```python
from build123d import *

# Parameters (mm, degrees)
F1_DEPTH = 6.35
F0_R     = 12.7
F2_DEPTH = 12.7
F3_DEPTH = 3.175
F4_R     = 3.175
F5_DEPTH = 180.976


with BuildPart() as f1:
    # F0 (on Top) → F1 (new body, symmetric)
    with BuildSketch(Plane.XY):
        with BuildLine():
            ThreePointArc((0, -31.75), (-31.75, 0), (0, 31.75))
            Line((0, 31.75), (0, 44.45))
            Line((0, 44.45), (-12.7, 44.45))
            Line((-12.7, 44.45), (-12.7, 31.75))
            Line((-12.7, 31.75), (-19.05, 31.75))
            ThreePointArc((-19.05, 31.75), (-37.291778, 15.423719), (-61.051302, 9.525))
            Line((-61.051302, 9.525), (-143.102955, 9.525))
            ThreePointArc((-143.102955, 9.525), (-150.147647, 10.521469), (-156.639598, 13.432692))
            ThreePointArc((-156.639598, 13.432692), (-151.201718, 7.671595), (-149.225, 0))
            ThreePointArc((-149.225, 0), (-151.201718, -7.671595), (-156.639598, -13.432692))
            ThreePointArc((-156.639598, -13.432692), (-150.147647, -10.521469), (-143.102955, -9.525))
            Line((-143.102955, -9.525), (-61.051302, -9.525))
            ThreePointArc((-61.051302, -9.525), (-37.291778, -15.423719), (-19.05, -31.75))
            Line((-19.05, -31.75), (-12.7, -31.75))
            Line((-12.7, -31.75), (-12.7, -44.45))
            Line((-12.7, -44.45), (0, -44.45))
            Line((0, -44.45), (0, -31.75))
        make_face()
        with BuildLine():
            ThreePointArc((-127, -6.35), (-133.35, 0), (-127, 6.35))
            Line((-127, 6.35), (-50.8, 6.35))
            ThreePointArc((-50.8, 6.35), (-44.45, 0), (-50.8, -6.35))
            Line((-50.8, -6.35), (-127, -6.35))
        make_face(mode=Mode.SUBTRACT)
    extrude(amount=F1_DEPTH, both=True)

    # F0 (on Top) → F2 (join, symmetric)
    with BuildSketch(Plane.XY):
        with BuildLine():
            ThreePointArc((-149.225, 0), (-151.201718, 7.671595), (-156.639598, 13.432692))
            ThreePointArc((-156.639598, 13.432692), (-180.975, 0), (-156.639598, -13.432692))
            ThreePointArc((-156.639598, -13.432692), (-151.201718, -7.671595), (-149.225, 0))
        make_face()
        with Locations((-165.1, 0)):
            Circle(F0_R, mode=Mode.SUBTRACT)
        with BuildLine():
            Line((0, 25.4), (0, 31.75))
            ThreePointArc((0, 31.75), (-31.75, 0), (0, -31.75))
            Line((0, -31.75), (0, -25.4))
            ThreePointArc((0, -25.4), (-25.4, 0), (0, 25.4))
        make_face()
    extrude(amount=F2_DEPTH, both=True)

    # F0 (on Top) → F3 (join, symmetric)
    with BuildSketch(Plane.XY):
        with BuildLine():
            Line((-50.8, 6.35), (-127, 6.35))
            ThreePointArc((-127, 6.35), (-133.35, 0), (-127, -6.35))
            Line((-127, -6.35), (-50.8, -6.35))
            ThreePointArc((-50.8, -6.35), (-44.45, 0), (-50.8, 6.35))
        make_face()
    extrude(amount=F3_DEPTH, both=True)

    # F4 (on face) → F5 (cut, through all)
    with BuildSketch(Plane.YZ):
        with Locations((-38.1, 0)):
            Circle(F4_R)
        with Locations((38.1, 0)):
            Circle(F4_R)
    extrude(amount=-F5_DEPTH, mode=Mode.SUBTRACT)


solid = f1.part
```
Check sheet for the modelled part. Datum: model origin and axes. Units: mm. A direction names the side the tool comes from. Round coordinates to 2 decimals unless told otherwise and drop trailing zeros. Order: outer loops, then holes, each group sorted by start corner. A loop starts at its lowest first (then second) coordinate and runs counter-clockwise, first axis right, second up. Notation, with made-up numbers: (27.25, 52) - (81.25, 52) arc R20 cw to (81.25, 58) - close; hole circle Ø1 at (83, 12). An arc over 180 degrees is marked (long way). Answer as CSV lines item,"result". Start each with the question number.
1) Section check A-A (z = 11). Record the cut outline in (x, y) (3 decimals).
2) Section check D-D (x = -63). Record the cut outline in (y, z) (3 decimals).
3) Draft check along Y on faces 1 (the face through (-25.394, -0.559, 0.178)), 2 (the face through (-6.26, -41.27, 0.14)), 3 (the face through (-6, -44.45, 0)), 4 (the face through (-12.7, 40, 3)). Enter one of: +Y half, -Y half, draft (parallel to the pull), parting line (faces both ways), or undercut.
4) Section check C-C (y = -38.1). Record the cut outline in (x, z) (3 decimals), then the cut area to 3 significant figures.
5) Tool access check on faces 5 (the face through (-150.24, -10.55, 0.09)), 6 (the face through (-31.742, 0.698, 9.569)), 7 (the face through (-102, 9.525, 0)), 8 (the face through (-16, -31.75, 0)). Record the directions out of +Z, -Z, +X, -X, +Y, -Y that give a thin tool (end or side, any length) a straight path to the whole face; none if there is none.
6) Depth check by flat-ended pin: pin 1 (2.5 mm diameter, centred on x = -75, z = 5.5, fed in from +Y) (3 decimals); pin 2 (3.5 mm diameter, centred on x = -86, z = -4.5, fed in from -Y) (3 decimals); pin 3 (10 mm diameter, centred on y = 37, z = -2.5, fed in from -X); pin 4 (23 mm diameter, centred on x = -165.1, y = 0, fed in from -Z). Enter the tip coordinate at first touch or a pass-through.
7) Section check B-B (x = -165.1). Record the cut outline in (y, z) (3 decimals), then the cut area to 3 significant figures.
8) Scan lines: probe 1 along Y at (x, z) = (-165.5, 3.5); probe 2 along Z at (x, y) = (-9.5, -38.1) (3 decimals); probe 3 along X at (y, z) = (-5, -6). Record each from-to range of solid material in increasing order.
Determined:
1,outline,"(-156.64, -13.433) arc R15.875 ccw to (-149.225, 0) arc R15.875 ccw to (-156.64, 13.433) arc R15.875 ccw (long way) to start; (0, -31.75) - (0, -25.4) arc R25.4 cw to (0, 25.4) - (0, 31.75) arc R31.75 ccw to start; hole circle Ø25.4 at (-165.1, 0)"
2,outline,"(-9.525, -6.35) - (-6.35, -6.35) - (-6.35, -3.175) - (6.35, -3.175) - (6.35, -6.35) - (9.525, -6.35) - (9.525, 6.35) - (6.35, 6.35) - (6.35, 3.175) - (-6.35, 3.175) - (-6.35, 6.35) - (-9.525, 6.35) - close"
3,face 1,"undercut"
3,face 2,"undercut"
3,face 3,"-Y half"
3,face 4,"draft"
4,outline,"(-12.7, -6.35) - (0, -6.35) - (0, -3.175) - (-12.7, -3.175) - close; (-12.7, 3.175) - (0, 3.175) - (0, 6.35) - (-12.7, 6.35) - close"
4,area,"80.6 mm^2"
5,face 5,"+Z, -Z, -Y"
5,face 6,"+Z"
5,face 7,"+Z, -Z, +Y"
5,face 8,"+Z, -Z, -X, -Y"
6,pin 1,"y = 9.525"
6,pin 2,"y = -9.525"
6,pin 3,"x = -12.7"
6,pin 4,"through"
7,outline,"(-15.875, -12.7) - (-12.7, -12.7) - (-12.7, 12.7) - (-15.875, 12.7) - close; (12.7, -12.7) - (15.875, -12.7) - (15.875, 12.7) - (12.7, 12.7) - close"
7,area,"161 mm^2"
8,probe 1,"-15.87 to -12.69, 12.69 to 15.87"
8,probe 2,"-6.35 to -3.175, 3.175 to 6.35"
8,probe 3,"-180.17 to -176.77, -153.43 to -130.91, -46.89 to -24.9"
